from build123d import *

# Parameters (mm, degrees)
SKETCH2_R           = 0.635
BOSS_EXTRUDE2_DEPTH = 0.635
SKETCH3_R           = 2.54
BOSS_EXTRUDE3_DEPTH = 3.302
SKETCH4_R           = 2.286
CUT_EXTRUDE1_DEPTH  = 3.302


with BuildPart() as part:
    # Sketch2 → Boss-Extrude2 (new body)
    with BuildSketch(Plane(origin=(0, 0, 0), x_dir=(1, 0, 0), z_dir=(0, 1, 0))):
        with BuildLine():
            Line((-10.16, -1.27), (-0.625230769, -2.461846154))
            ThreePointArc((-0.625230769, -2.461846154), (0, -2.54), (0.625230769, -2.461846154))
            Line((0.625230769, -2.461846154), (10.16, -1.27))
            ThreePointArc((10.16, -1.27), (11.43, 0), (10.16, 1.27))
            Line((10.16, 1.27), (0.625230769, 2.461846154))
            ThreePointArc((0.625230769, 2.461846154), (0, 2.54), (-0.625230769, 2.461846154))
            Line((-0.625230769, 2.461846154), (-10.16, 1.27))
            ThreePointArc((-10.16, 1.27), (-11.43, 0), (-10.16, -1.27))
        make_face()
        with Locations((5.08, 0)):
            Circle(SKETCH2_R, mode=Mode.SUBTRACT)
        with Locations((10.16, 0)):
            Circle(SKETCH2_R, mode=Mode.SUBTRACT)
        with Locations((-10.16, 0)):
            Circle(SKETCH2_R, mode=Mode.SUBTRACT)
        with Locations((-5.08, 0)):
            Circle(SKETCH2_R, mode=Mode.SUBTRACT)
    extrude(amount=BOSS_EXTRUDE2_DEPTH)

    # Sketch3 → Boss-Extrude3 (add)
    with BuildSketch(Plane.XZ):
        Circle(SKETCH3_R)
    extrude(amount=BOSS_EXTRUDE3_DEPTH)

    # Sketch4 → Cut-Extrude1 (cut)
    with BuildSketch(Plane(origin=(0, -3.302, 0), x_dir=(-1, 0, 0), z_dir=(0, -1, 0))):
        Circle(SKETCH4_R)
    extrude(amount=-CUT_EXTRUDE1_DEPTH, mode=Mode.SUBTRACT)


solid = part.part
Read the model definition and answer for the solid it produces. Units are mm, in the model's axes. A direction names the side the tool comes from. Give positions to 0.01 mm unless a question says otherwise; leave off trailing zeros. Write each loop counter-clockwise with the first axis right and the second up, starting at its lowest first coordinate (ties: lowest second). Pieces come first, ordered by that corner, then holes. Notation, with made-up numbers: (19, -22.5) -> (31, -22.5) arc R24 cw to (31, -5.5) -> close; hole circle Ø1 at (71, 7). An arc over 180 degrees is marked (long way). Answer as a JSON object with one key per item and string values. Group by question number.
1) Find section B-B (y = -2.4). Write down the section's boundary in (x, z), and give its area (3 significant figures).
2) Consider L1, parallel to X at y = 0.25, z = 0 (3 decimals); L2, parallel to X at y = -1.5, z = 0. Determine where each line is inside the solid, lowest interval first. Write a range as from..to.
3) The mould has two halves that part along Z. Classify faces 3 (the flat face through (6, 0, 0)), 4 (the cylindrical face through (-10.794, 0.313, -0.028)), 5 (the cylindrical face through (-11.43, 0.31, -0.03)), 6 (the cylindrical face through (-4.49, 0.31, 0.24)): +Z half, -Z half, draft (parallel to the pull), parting line (faces both ways), or undercut.
4) A tool of negligible diameter and unlimited length cuts with its end or side. For faces 1 (the cylindrical face through (11.43, 0.31, 0.03)), 2 (the cylindrical face through (0.5, -1.67, 2.23)), from which of +Z, -Z, +X, -X, +Y, -Y can it reach the whole face along a straight path? Write none if from no direction.
5) Find section A-A (x = 5.08). Write down the section's boundary in (y, z) (3 decimals).
6) Find section D-D (x = 8). Write down the section's boundary in (y, z) (3 decimals).
7) Find section C-C (z = 0.3). Write down the section's boundary in (x, y) (3 decimals).
8) Each of these flat-tipped pins is pushed along its axis until it touches: P1, Ø2, axis at x = -5.08, z = 0, coming from the +Y side (3 decimals); P2, Ø1.5, axis at x = -5.5, z = -0.5, coming from the -Y side. Where does it stop, or does it pass through?
Values follow:
{
 "1": {"outline": "circle Ø5.08 at (0, 0); hole circle Ø4.57 at (0, 0)", "area": "3.85 mm2"},
 "2": {"L1": "x = -11.43..-10.795, -9.525..-5.715, -4.445..4.445, 5.715..9.525, 10.795..11.43", "L2": "x = -2.54..-2.29, 2.29..2.54"},
 "3": {"face 3": "draft", "face 4": "undercut", "face 5": "parting line", "face 6": "undercut"},
 "4": {"face 1": "+X, +Y, -Y", "face 2": "-Y"},
 "5": {"outline": "(0, -1.905) -> (0.635, -1.905) -> (0.635, -0.635) -> (0, -0.635) -> close; (0, 0.635) -> (0.635, 0.635) -> (0.635, 1.905) -> (0, 1.905) -> close"},
 "6": {"outline": "(0, -1.54) -> (0.635, -1.54) -> (0.635, 1.54) -> (0, 1.54) -> close"},
 "7": {"outline": "(-11.394, 0) -> (-10.72, 0) -> (-10.72, 0.635) -> (-11.394, 0.635) -> close; (-9.6, 0) -> (-5.64, 0) -> (-5.64, 0.635) -> (-9.6, 0.635) -> close; (-4.52, 0) -> (-2.522, 0) -> (-2.522, -3.302) -> (-2.266, -3.302) -> (-2.266, 0) -> (2.266, 0) -> (2.266, -3.302) -> (2.522, -3.302) -> (2.522, 0) -> (4.52, 0) -> (4.52, 0.635) -> (-4.52, 0.635) -> close; (5.64, 0) -> (9.6, 0) -> (9.6, 0.635) -> (5.64, 0.635) -> close; (10.72, 0) -> (11.394, 0) -> (11.394, 0.635) -> (10.72, 0.635) -> close"},
 "8": {"P1": "stops at y = 0.635", "P2": "stops at y = 0"}
}
